from build123d import *

# Parameters (mm, degrees)
SKETCH2_R           = 1.5
BOSS_EXTRUDE1_DEPTH = 2.62


with BuildPart() as part:
    # Sketch2 → Boss-Extrude1 (new body)
    with BuildSketch(Plane.XY):
        with BuildLine():
            Line((-0.779366827, 34.5), (0.779366827, 34.5))
            ThreePointArc((0.779366827, 34.5), (3.503665988, 33.428855422), (4.768906011, 30.789097042))
            Line((4.768906011, 30.789097042), (7, 0))
            Line((7, 0), (4.5, -9))
            Line((4.5, -9), (-4.5, -9))
            Line((-4.5, -9), (-7, 0))
            Line((-7, 0), (-4.768906011, 30.789097042))
            ThreePointArc((-4.768906011, 30.789097042), (-3.503665988, 33.428855422), (-0.779366827, 34.5))
        make_face()
        Circle(SKETCH2_R, mode=Mode.SUBTRACT)
        with Locations((0, 19.1)):
            Circle(SKETCH2_R, mode=Mode.SUBTRACT)
        with Locations((0, 24.3)):
            Circle(SKETCH2_R, mode=Mode.SUBTRACT)
        with Locations((0, 29.5)):
            Circle(SKETCH2_R, mode=Mode.SUBTRACT)
    extrude(amount=BOSS_EXTRUDE1_DEPTH)


solid = part.part
Could you check a few things on this model? Use its own coordinates, in mm. Round coordinates to 2 decimals unless told otherwise and drop trailing zeros. Write each loop counter-clockwise with the first axis right and the second up, starting at its lowest first coordinate (ties: lowest second). Pieces come first, ordered by that corner, then holes. Notation, with made-up numbers: (-15.5, -17) -> (24.5, -17) arc R17 ccw to (24.5, 1) -> close; hole circle Ø4 at (49.25, 6.5). An arc over 180 degrees is marked (long way). Use a Markdown table: item, result.
1. We'd pull the mould along X, two halves only. Please class faces 1 (the face through (-3.534, 33.4, 1.292)), 2 (the face through (0, -9, 1)), 3 (the face through (-0.325, 22.836, 1.292)): +X half, -X half, draft (parallel to the pull), parting line (faces both ways), or undercut.
Answer key:
| item | result |
|---|---|
| face 1 | -X half |
| face 2 | draft |
| face 3 | undercut |
2. If we section it at A-A (z = 1.2): List the corners of the cut face in (x, y) for me, then the cut area to 3 significant figures.
Answer key:
| item | result |
|---|---|
| outline | (-7, 0) -> (-4.5, -9) -> (4.5, -9) -> (7, 0) -> (4.77, 30.79) arc R4 ccw to (0.78, 34.5) -> (-0.78, 34.5) arc R4 ccw to (-4.77, 30.79) -> close; hole circle Ø3 at (0, 0); hole circle Ø3 at (0, 19.1); hole circle Ø3 at (0, 24.3); hole circle Ø3 at (0, 29.5) |
| area | 466 mm^2 |
3. For pin 1 Ø1.8 at (x, y) = (0, 29.5) entering from +Z; pin 2 Ø1.5 at (x, z) = (-2, 0.5) entering from +Y, each with a flat end and sliding along its axis, tell me the tip position at first contact or that it passes through.
Answer key:
| item | result |
|---|---|
| pin 1 | passes through |
| pin 2 | stops at y = 34.47 |
4. Please list where these lines run through material, in increasing order: probe 1 along Y at (x, z) = (0, 1.6); probe 2 along Y at (x, z) = (-1.25, 2.45); probe 3 along X at (y, z) = (28.5, 0.9).
Answer key:
| item | result |
|---|---|
| probe 1 | y = -9 to -1.5, 1.5 to 17.6, 20.6 to 22.8, 25.8 to 28, 31 to 34.5 |
| probe 2 | y = -9 to -0.83, 0.83 to 18.27, 19.93 to 23.47, 25.13 to 28.67, 30.33 to 34.47 |
| probe 3 | x = -4.93 to -1.12, 1.12 to 4.93 |
5. If we section it at D-D (y = -4.5): List the corners of the cut face in (x, z) for me.
Answer key:
| item | result |
|---|---|
| outline | (-5.75, 0) -> (5.75, 0) -> (5.75, 2.62) -> (-5.75, 2.62) -> close |
6. If we section it at B-B (x = 0): List the corners of the cut face in (y, z) for me.
Answer key:
| item | result |
|---|---|
| outline | (-9, 0) -> (-1.5, 0) -> (-1.5, 2.62) -> (-9, 2.62) -> close; (1.5, 0) -> (17.6, 0) -> (17.6, 2.62) -> (1.5, 2.62) -> close; (20.6, 0) -> (22.8, 0) -> (22.8, 2.62) -> (20.6, 2.62) -> close; (25.8, 0) -> (28, 0) -> (28, 2.62) -> (25.8, 2.62) -> close; (31, 0) -> (34.5, 0) -> (34.5, 2.62) -> (31, 2.62) -> close |
7. If we section it at C-C (y = 19.1): List the corners of the cut face in (x, z) for me, then the cut area to 3 significant figures.
Answer key:
| item | result |
|---|---|
| outline | (-5.62, 0) -> (-1.5, 0) -> (-1.5, 2.62) -> (-5.62, 2.62) -> close; (1.5, 0) -> (5.62, 0) -> (5.62, 2.62) -> (1.5, 2.62) -> close |
| area | 21.6 mm^2 |
